The model under review builds one solid part; all positions refer to its coordinate system, in mm. Face numbers are marked on the shaded views. A direction names the side the tool comes from. Round coordinates to 2 decimals unless told otherwise and drop trailing zeros. Order: outer loops, then holes, each group sorted by start corner. A loop starts at its lowest first (then second) coordinate and runs counter-clockwise, first axis right, second up. Notation, with made-up numbers: M 79.5,62 L 125.5,62 A21 ccw 125.5,90 Z; hole C -22,-14 d8. An arc over 180 degrees is marked long. Answer as a JSON object with one key per item and string values. Group by question number.
1. Machinability: for the marked faces 1, 2, 3, 4 and 5, which of the approach directions +Z, -Z, +X, -X, +Y, -Y give a long, thin tool a straight path to every point of the face, cutting with its end or side? Answer none if there is none.
2. Mouldability with a two-part tool opening along X and no side actions: class the marked faces 6, 7 and 8 as released by +X, released by -X, zero draft, split by the parting line, or undercut.
3. To check wall thickness, follow probe 1 along Y at (x, z) = (37.5, 7.5); probe 2 along X at (y, z) = (-15, 6.75); probe 3 along Z at (x, y) = (31.5, 9). State the ranges of each line that lie inside material, in increasing order. Write a range as [from, to].
4. Add section A-A on z = 4. State the section outline as (x, y) points, and give its area (3 significant figures).
5. Add section D-D on z = 27. State the section outline as (x, y) points.
6. Add section C-C on x = -31. State the section outline as (y, z) points, and give its area (3 significant figures).
7. Add section B-B on z = 34. State the section outline as (x, y) points, and give its area (3 significant figures).
8. Clearance check with flat-ended pins moving along their axes: P1, Ø20, axis at x = 13.5, z = 27, coming from the -Y side; P2, Ø4.5, axis at y = 0, z = 7.5, coming from the -X side; P3, Ø14.5, axis at x = 10, z = 24, coming from the +Y side. State where each tip first meets the part, or that it passes through.
Autodesk Inventor part; units mm, degrees
ref_plane "YZ Plane" through (0, 0, 0) normal (1, 0, 0) x (0, 1, 0)
ref_plane "XZ Plane" through (0, 0, 0) normal (0, 1, 0) x (-1, 0, 0)
ref_plane "XY Plane" through (0, 0, 0) normal (0, 0, 1) x (1, 0, 0)
sketch "Эскиз1" plane through (0, 0, 0) normal (0, 0, 1) x (1, 0, 0)
  line L0 (-47.5, -25) -> (47.5, -25)
  line L1 (47.5, -25) -> (47.5, 25)
  line L2 (47.5, 25) -> (-47.5, 25)
  line L3 (-47.5, 25) -> (-47.5, -25)
  line L4 (-47.5, -25) -> (47.5, 25) construction
  line L5 (47.5, -25) -> (-47.5, 25) construction
  point P0 (0, 0)
  dimension "d0" = 95
  dimension "d1" = 50
extrude "Выдавливание1" add sketch "Эскиз1" along normal blind 15
sketch "Эскиз2" plane through (-47.5, -25, 0) normal (-1, 0, 0) x (0, 0, 1)
  point P0 (0, 25)
sketch "Эскиз3" plane through (-47.5, -25, 0) normal (-1, 0, 0) x (0, 0, 1)
  line L0 (15, 0) -> (15, 50)
  line L1 (0, 35) -> (15, 35)
  line L2 (15, 35) -> (15, 15)
  line L3 (15, 15) -> (0, 15)
  line L4 (0, 15) -> (0, 35)
  line L5 (0, 25) -> (15, 25)
  dimension "d4" = 20
extrude "Выдавливание2" cut sketch "Эскиз3" against normal blind 15
fillet "Сопряжение1" radius 10 1 edges at (47.5, 25, 7.5)
fillet "Сопряжение2" radius 10 1 edges at (47.5, -25, 7.5)
sketch "Эскиз4" plane through (0, 0, 15) normal (0, 0, 1) x (1, 0, 0)
  line L0 (0, 0) -> (47.5, 0)
  line L1 (47.5, -15) -> (47.5, 15)
  line L2 (-47.5, 25) -> (-47.5, 10)
  point P0 (37.5, 15)
  point P1 (37.5, -15)
  dimension "d9" = 30
  dimension "d10" = 85
hole "Отверстие1" at (37.5, 15, 15) at (37.5, -15, 15) direction (0, 0, -1) diameter 10 end through all
sketch "Эскиз5" plane through (0, 0, 15) normal (0, 0, 1) x (1, 0, 0)
  circle A0 centre (-7.5, 0) radius 13
  line L0 (-47.5, 25) -> (-47.5, 10)
  point P0 (0, 0)
  dimension "d18" = 26
  dimension "d19" = 40
extrude "Выдавливание3" add sketch "Эскиз5" along normal blind 25
sketch "Эскиз6" plane through (-7.5, 0, 40) normal (0, 0, 1) x (1, 0, 0)
  point P0 (7.5, 0)
  point P1 (0, 0)
hole "Отверстие2" at (-7.5, 0, 40) direction (0, 0, -1) diameter 16 depth 30 tip angle 118
chamfer "Фаска1" distance 2 angle 45 1 edges at (-7.5, 8, 40)
sketch "Эскиз7" plane through (0, 0, 15) normal (0, 0, 1) x (1, 0, 0)
  point P0 (0, 0)
sketch "Эскиз8" plane through (0, 0, 0) normal (0, 1, 0) x (-1, 0, 0)
  line L0 (20.5, 40) -> (-5.5, 40)
  line L1 (0, 40) -> (-11.4909, 40)
  line L2 (-11.4909, 40) -> (-5.5, 35)
  line L3 (-5.5, 15) -> (-5.5, 40)
  line L4 (-5.5, 35) -> (-22.5, 15)
  line L5 (47.5, 0) -> (47.5, 15)
  line L6 (-22.5, 15) -> (47.5, 15)
  line L7 (-5.5, 35) -> (-1.25, 40)
  line L8 (17.5, 40) -> (-2.5, 40)
  line L9 (-2.5, 40) -> (-0.5, 38)
  line L10 (-1.8243, 39.3243) -> (-1.8243, 15)
  line L11 (-37.5, 15) -> (47.5, 15)
  point P0 (0, 0)
  dimension "d32" = 70
  dimension "d33" = 5
extrude "Выдавливание4" add sketch "Эскиз8" along normal mid plane 10 contours L10 L6 L3 L7 | L3 L6 L4
properties part number "Основание"
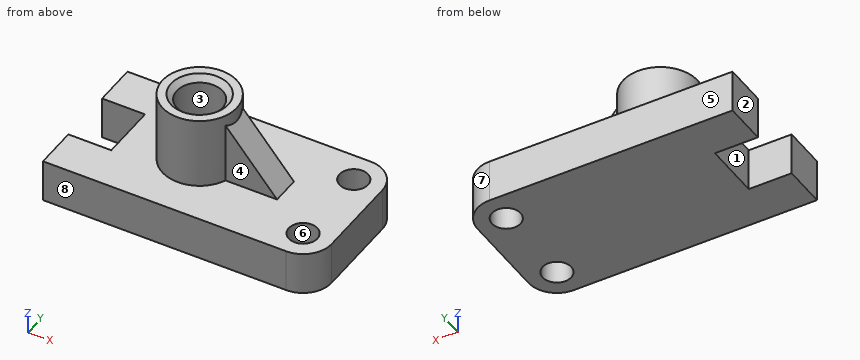
Recorded:
{
 "1": {"face 1": "+Z, -Z, -X", "face 2": "+Z, -Z, -X, +Y, -Y", "face 3": "+Z", "face 4": "+Z, +X, -Y", "face 5": "+Z, -Z, +X, -X, +Y"},
 "2": {"face 6": "undercut", "face 7": "released by +X", "face 8": "zero draft"},
 "3": {"probe 1": "y = [-25, -20], [-10, 10], [20, 25]", "probe 2": "x = [-47.5, 32.5], [42.5, 47.5]", "probe 3": "z = [0, 15]"},
 "4": {"outline": "M -47.5,-25 L 37.5,-25 A10 ccw 47.5,-15 L 47.5,15 A10 ccw 37.5,25 L -47.5,25 L -47.5,10 L -32.5,10 L -32.5,-10 L -47.5,-10 Z; hole C 37.5,-15 d10; hole C 37.5,15 d10", "area": "4,250 mm²"},
 "5": {"outline": "M 4.5,-5 L 12.3,-5 L 12.3,5 L 4.5,5 A13 ccw long Z; hole C -7.5,0 d16"},
 "6": {"outline": "M -25,0 L 25,0 L 25,15 L -25,15 Z", "area": "750 mm²"},
 "7": {"outline": "M 4.5,-5 L 6.35,-5 L 6.35,5 L 4.5,5 A13 ccw long Z; hole C -7.5,0 d16", "area": "342 mm²"},
 "8": {"P1": "stops at y = -6.93", "P2": "stops at x = -32.5", "P3": "stops at y = 8"}
}
